```python
from build123d import *

# Parameters (mm, degrees)
F1_DEPTH = 19.05


with BuildPart() as f1:
    # F0 (on Front) → F1 (new body)
    with BuildSketch(Plane.XZ):
        Polygon((-163.861383, 222.770982), (-163.861383, -142.354018), (-62.261383, -142.354018), (-62.261383, 222.770982), (-113.061383, 222.770982), align=None)
        with BuildLine():
            ThreePointArc((-152.063083, 175.027341), (-133.626353, 184.734933), (-113.061383, 188.08641))
            ThreePointArc((-113.061383, 188.08641), (-92.496414, 184.734933), (-74.059683, 175.027341))
            Line((-74.059683, 175.027341), (-74.059683, -7.878059))
            ThreePointArc((-74.059683, -7.878059), (-113.061383, -20.937129), (-152.063083, -7.878059))
            Line((-152.063083, -7.878059), (-152.063083, 175.027341))
        make_face(mode=Mode.SUBTRACT)
    extrude(amount=F1_DEPTH)


solid = f1.part
```
The model under review builds one solid part; all positions refer to its coordinate system, in mm. A direction names the side the tool comes from. Round coordinates to 2 decimals unless told otherwise and drop trailing zeros. Loops run counter-clockwise (first coordinate to the right, second up) from the corner with the lowest first, then second, coordinate; pieces in that order, holes last. Notation, with made-up numbers: (7, 85.25) -> (26, 85.25) arc R27 cw to (26, 107.25) -> close; hole circle Ø10 at (-17.5, -15). An arc over 180 degrees is marked (long way). Answer in a Markdown table with one row per item.
1) Tool access review of faces 5 (the flat face through (-112, -9, 222.771)), 6 (the flat face through (-152.063, -9, 82)): name each direction out of +Z, -Z, +X, -X, +Y, -Y from which nothing blocks a thin tool from reaching the whole face with its end or side.
Taken from the geometry:
| item | result |
|---|---|
| face 5 | +Z, +X, -X, +Y, -Y |
| face 6 | +Y, -Y |
2) Wall thickness on line 1 along X through (y, z) = (-2.25, 146); line 2 along Z through (x, y) = (-78, -18); line 3 along Z through (x, y) = (-99, -5): over which ranges is each line inside the solid? List them lowest first.
Taken from the geometry:
| item | result |
|---|---|
| line 1 | x = -163.86 to -152.06, -74.06 to -62.26 |
| line 2 | z = -142.35 to -10.63, 177.78 to 222.77 |
| line 3 | z = -142.35 to -19.39, 186.54 to 222.77 |
3) Consider section A-A, the plane z = 78. Write out the cut boundary in (x, y).
Taken from the geometry:
| item | result |
|---|---|
| outline | (-163.86, -19.05) -> (-152.06, -19.05) -> (-152.06, 0) -> (-163.86, 0) -> close; (-74.06, -19.05) -> (-62.26, -19.05) -> (-62.26, 0) -> (-74.06, 0) -> close |
4) Consider section C-C, the plane y = -10. Write out the cut boundary in (x, z), plus the area to 3 significant figures.
Taken from the geometry:
| item | result |
|---|---|
| outline | (-163.86, -142.35) -> (-62.26, -142.35) -> (-62.26, 222.77) -> (-163.86, 222.77) -> close; hole (-152.06, -7.88) arc R64.77 ccw to (-74.06, -7.88) -> (-74.06, 175.03) arc R64.77 ccw to (-113.06, 188.09) arc R64.77 ccw to (-152.06, 175.03) -> close |
| area | 21,400 mm² |
5) Draft analysis for pull direction X (two halves, no side actions). For faces 1 (the flat face through (-163.861, -9, 43)), 2 (the flat face through (-159, -19.05, 2)), 3 (the flat face through (-74.06, -9, 85)), 4 (the flat face through (-62.261, -9, 38)), state which applies: pulls with the +X half, pulls with the -X half, needs draft (parallel to the pull), parting line crosses it, or undercut.
Taken from the geometry:
| item | result |
|---|---|
| face 1 | pulls with the -X half |
| face 2 | needs draft |
| face 3 | undercut |
| face 4 | pulls with the +X half |
6) Consider section B-B, the plane x = -148. Write out the cut boundary in (y, z).
Taken from the geometry:
| item | result |
|---|---|
| outline | (-19.05, -142.35) -> (0, -142.35) -> (0, -10.71) -> (-19.05, -10.71) -> close; (-19.05, 177.85) -> (0, 177.85) -> (0, 222.77) -> (-19.05, 222.77) -> close |
